Input: part model. Units: mm. Frame: model coordinates. Round coordinates to 2 decimals unless told otherwise and drop trailing zeros. Loops run counter-clockwise (first coordinate to the right, second up) from the corner with the lowest first, then second, coordinate; pieces in that order, holes last.
1) Section A-A, the plane x = 0. Return loops of the section in (y, z) (3 decimals), and give its area (3 significant figures).
2) Ray query, line 1 along Y through (x, z) = (16, 2) (3 decimals); line 2 along X through (y, z) = (-0.5, 3); line 3 along X through (y, z) = (0.75, 3). Return the intervals inside material, ascending.
3) Draft query along X for faces 1 (the face through (-19.9, 0.1, 3.8)), 2 (the face through (0, -3.9, 4)), 3 (the face through (-13.687, 0.728, 3.845)). Return one class per face: pulls with the +X half, pulls with the -X half, needs draft (parallel to the pull), parting line crosses it, or undercut.
4) Section B-B, the plane z = 3. Return loops of the section in (x, y) (3 decimals).
5) First-contact query: pin 1 (1.5 mm diameter, centred on y = 3, z = 4.5, fed in from +X). Flat tip, straight axial feed; report the tip coordinate or a pass-through.
6) Section C-C, the plane y = 0. Return loops of the section in (x, z) (3 decimals).
7) Section D-D, the plane x = -16.5. Return loops of the section in (y, z), and give its area (3 significant figures).
from build123d import *

# Parameters (mm, degrees)
F0_R     = 2.425
F1_DEPTH = 7.8
F2_R     = 2.425
F3_DEPTH = 7.8


with BuildPart() as f1:
    # F0 (on Top) → F1 (new body)
    with BuildSketch(Plane.XY):
        with BuildLine():
            ThreePointArc((16, -3.9), (19.9, 0), (16, 3.9))
            Line((16, 3.9), (-16, 3.9))
            ThreePointArc((-16, 3.9), (-19.9, 0), (-16, -3.9))
            Line((-16, -3.9), (16, -3.9))
        make_face()
        with Locations((-16, 0)):
            Circle(F0_R, mode=Mode.SUBTRACT)
        Circle(F0_R, mode=Mode.SUBTRACT)
        with Locations((16, 0)):
            Circle(F0_R, mode=Mode.SUBTRACT)
    extrude(amount=F1_DEPTH)

    # F2 (on face) → F3 (join)
    with BuildSketch(Plane.XZ.offset(3.9)):
        with Locations((-8, 3.9)):
            Circle(F2_R)
        with BuildLine():
            ThreePointArc((10.425, 3.9), (8, 6.325), (5.575, 3.9))
            ThreePointArc((5.575, 3.9), (8, 1.475), (10.425, 3.9))
        make_face()
    extrude(amount=-F3_DEPTH)


solid = f1.part
Final values:
1. outline: (-3.9, 0) - (-2.425, 0) - (-2.425, 7.8) - (-3.9, 7.8) - close; (2.425, 0) - (3.9, 0) - (3.9, 7.8) - (2.425, 7.8) - close
1. area: 23.0 mm2
2. line 1: y = -3.9 to -2.425, 2.425 to 3.9
2. line 2: x = -19.87 to -18.37, -13.63 to -2.37, 2.37 to 13.63, 18.37 to 19.87
2. line 3: x = -19.83 to -18.31, -13.69 to -2.31, 2.31 to 13.69, 18.31 to 19.83
3. face 1: pulls with the -X half
3. face 2: needs draft
3. face 3: undercut
4. outline: (-16, -3.9) - (16, -3.9) arc R3.9 ccw to (16, 3.9) - (-16, 3.9) arc R3.9 ccw to start; hole circle Ø4.85 at (-16, 0); hole circle Ø4.85 at (0, 0); hole circle Ø4.85 at (16, 0)
5. pin 1: stops at x = 19.19
6. outline: (-19.9, 0) - (-18.425, 0) - (-18.425, 7.8) - (-19.9, 7.8) - close; (-13.575, 0) - (-2.425, 0) - (-2.425, 7.8) - (-13.575, 7.8) - close; (2.425, 0) - (13.575, 0) - (13.575, 7.8) - (2.425, 7.8) - close; (18.425, 0) - (19.9, 0) - (19.9, 7.8) - (18.425, 7.8) - close
7. outline: (-3.87, 0) - (-2.37, 0) - (-2.37, 7.8) - (-3.87, 7.8) - close; (2.37, 0) - (3.87, 0) - (3.87, 7.8) - (2.37, 7.8) - close
7. area: 23.3 mm2
